Could you check a few things on this drawing? It's one solid part, dimensions in mm from its lowest x, y, z. Give positions to 0.01 mm unless a question says otherwise; leave off trailing zeros. Loops run counter-clockwise (first coordinate to the right, second up) from the corner with the lowest first, then second, coordinate; pieces in that order, holes last. Notation, with made-up numbers: (88, -25) - (95, -25) arc R18 ccw to (95, -11) - close; hole circle Ø7 at (76.25, 21). An arc over 180 degrees is marked (long way). Use a Markdown table: item, result.
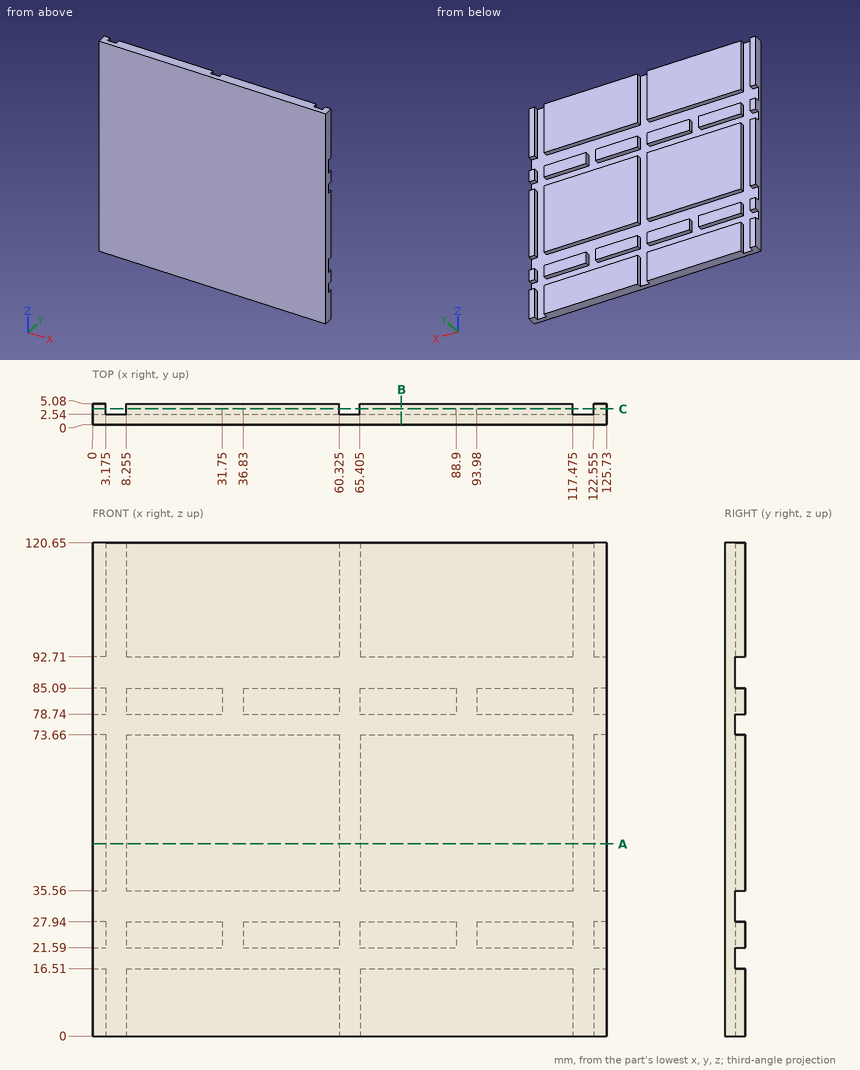
(1) Will this pin go through, and if not, where does the flat tip stop? pin 1 (2 mm diameter, centred on x = 91, z = 21, fed in from +Y).
A:
| item | result |
|---|---|
| pin 1 | y = 2.54 |
(2) If I drill on line 1 (Z direction, x = 109.5, y = 2.75); line 2 (Z direction, x = 32, y = 3.55); line 3 (X direction, y = 4.85, z = 25) (3 decimals), over which ranges is the centre line in solid material (lowest first)?
A:
| item | result |
|---|---|
| line 1 | 0 to 16.51, 21.59 to 27.94, 35.56 to 73.66, 78.74 to 85.09, 92.71 to 120.65 |
| line 2 | 0 to 16.51, 35.56 to 73.66, 92.71 to 120.65 |
| line 3 | 0 to 3.175, 8.255 to 31.75, 36.83 to 60.325, 65.405 to 88.9, 93.98 to 117.475, 122.555 to 125.73 |
(3) Suppose I cut it at C-C on y = 3.9. Count the separate pieces of the cut face and the enclosed holes in it, plus the area to 3 significant figures.
A:
| item | result |
|---|---|
| separate pieces | 24 |
| enclosed holes | 0 |
| area | 10,400 mm2 |
(4) Suppose I cut it at A-A on z = 47. Write out the boundary of the cut face in (x, y) (3 decimals).
A:
| item | result |
|---|---|
| outline | (0, 0) - (125.73, 0) - (125.73, 5.08) - (122.555, 5.08) - (122.555, 2.54) - (117.475, 2.54) - (117.475, 5.08) - (65.405, 5.08) - (65.405, 2.54) - (60.325, 2.54) - (60.325, 5.08) - (8.255, 5.08) - (8.255, 2.54) - (3.175, 2.54) - (3.175, 5.08) - (0, 5.08) - close |
(5) Suppose I cut it at B-B on x = 75.5. Write out the boundary of the cut face in (y, z), plus the area to 3 significant figures.
A:
| item | result |
|---|---|
| outline | (0, 0) - (5.08, 0) - (5.08, 16.51) - (2.54, 16.51) - (2.54, 21.59) - (5.08, 21.59) - (5.08, 27.94) - (2.54, 27.94) - (2.54, 35.56) - (5.08, 35.56) - (5.08, 73.66) - (2.54, 73.66) - (2.54, 78.74) - (5.08, 78.74) - (5.08, 85.09) - (2.54, 85.09) - (2.54, 92.71) - (5.08, 92.71) - (5.08, 120.65) - (0, 120.65) - close |
| area | 548 mm2 |
